The listing builds one solid part. Answer for the finished solid, in the listing's coordinates (mm). A direction names the side the tool comes from. Coordinates: 2 decimals unless noted, no trailing zeros. Loops run counter-clockwise (first coordinate to the right, second up) from the corner with the lowest first, then second, coordinate; pieces in that order, holes last. Notation, with made-up numbers: (58.5, 45) - (63.5, 45) arc R17 ccw to (63.5, 49) - close; hole circle Ø6 at (77, -16). An arc over 180 degrees is marked (long way). Write each question's results on one line, items separated by ' | '. Start each with the question number.
(1) Determine the mould class of faces 1 (the flat face through (3, -6, 0)), 2 (the cylindrical face through (-0.104, 12.12, 18.001)), 3 (the cylindrical face through (-10.54, 27.12, 35.69)) for opening direction Y: released by +Y, released by -Y, zero draft, split by the parting line, or undercut.
(2) For faces 4 (the flat face through (-17, -3, 38.1)), 5 (the cylindrical face through (15.023, -3.79, 17.24)), determine the directions among +Z, -Z, +X, -X, +Y, -Y from which every point of the face is accessible in a straight line to the end or side of a thin tool.
(3) Consider line 1 (X direction, y = 2.5, z = 30.5); line 2 (Y direction, x = -14.5, z = 15); line 3 (Y direction, x = 3, z = 32.5). Determine where each line is inside the solid, lowest interval first. Write a range as from..to.
(4) Given pin 1 Ø4 at (x, z) = (0.5, 13.5) entering from -Y; pin 2 Ø12 at (y, z) = (-9, 9) entering from -X; pin 3 Ø15 at (x, y) = (-13.5, -4) entering from -Z; pin 4 Ø5 at (x, y) = (-20, 22.5) entering from -Z, each flat-ended and moving along its own axis, determine where each tip first touches the part or whether it passes through.
(5) Find section A-A on z = 10. Determine the outline of the cut face in (x, y) (3 decimals), then the cut area to 3 significant figures.
Autodesk Inventor part; units mm, degrees
ref_plane "YZ Plane" through (0, 0, 0) normal (1, 0, 0) x (0, 1, 0)
ref_plane "XZ Plane" through (0, 0, 0) normal (0, 1, 0) x (-1, 0, 0)
ref_plane "XY Plane" through (0, 0, 0) normal (0, 0, 1) x (1, 0, 0)
sketch "Sketch1" plane through (0, 0, 0) normal (0, 0, 1) x (1, 0, 0)
  circle A0 centre (-5.0854, 2.5427) radius 10.795
  circle A1 centre (-5.0854, 2.5427) radius 21.082
  point P0 (0, 0)
  dimension "d0" = 21.59
  dimension "d1" = 42.164
extrude "Extrusion1" add sketch "Sketch1" along normal blind 38.1
ref_plane "Work Plane1" through (-5.0854, 2.5427, 33.3375) normal (0, 0, 1) x (1, 0, 0)
sketch "Sketch2" plane through (-5.0854, 2.5427, 33.3375) normal (0, 0, 1) x (1, 0, 0)
  circle A0 centre (0, 0) radius 10.795
  circle A1 centre (0, 0) radius 25.1734
  point P0 (5.0854, -2.5427)
extrude "Extrusion2" add sketch "Sketch2" along normal blind 4.7625
fillet "Fillet1" radius 1.5875 2 edges at (-15.8804, 2.5427, 38.1) (-26.1674, 2.5427, 0)
properties part number "pvcconnector"
Values:
1) face 1: zero draft | face 2: undercut | face 3: split by the parting line
2) face 4: +Z, +X, -X, +Y, -Y | face 5: -Z
3) line 1: x = -26.17..-15.88, 5.71..16 | line 2: y = -16.32..-2.74, 7.82..21.41 | line 3: y = -16.93..-4.61, 9.7..22.01
4) pin 1: stops at y = -18.23 | pin 2: stops at x = -25.43 | pin 3: stops at z = 0 | pin 4: stops at z = 33.34
5) outline: circle Ø42.164 at (-5.085, 2.543); hole circle Ø21.59 at (-5.085, 2.543) | area: 1,030 mm²
